Study the drawing (mm; zero at the part's minimum x, y, z) and answer. A direction names the side the tool comes from. Round coordinates to 2 decimals unless told otherwise and drop trailing zeros. Loops run counter-clockwise (first coordinate to the right, second up) from the corner with the lowest first, then second, coordinate; pieces in that order, holes last. Notation, with made-up numbers: M 28,-29 L 78,-29 A21 cw 78,-12 Z; hole C 52,-4.5 d2. An arc over 180 degrees is marked long. Put each result on its own line as item: value. Start each with the question number.
(1) Which of the six approach directions +Z, -Z, +X, -X, +Y, -Y give full straight-line access (tool end or side, diameter ignored) to the marked faces 1 and 2?
(2) Section B-B, the plane x = 28.5 is taken. Determine the outline of the cut face in (y, z).
(3) Section A-A, the plane y = 1.5 is taken. Determine the outline of the cut face in (x, z).
(4) Section C-C, the plane z = 6 is taken. Determine the outline of the cut face in (x, y).
(5) Determine the mould class of the marked faces 3, 4, 5 and 6 for opening direction X: released by +X, released by -X, zero draft, split by the parting line, or undercut.
(6) Section D-D, the plane y = 9 is taken. Determine the outline of the cut face in (x, z), then the cut area to 3 significant figures.
(7) Straight lines are drawn through the part: line 1 (X direction, y = 9.75, z = 41.9); line 2 (Z direction, x = 28.5, y = 10.35); line 3 (X direction, y = 5, z = 37). For each, find the intervals that lie inside material, in ascending order.
(8) Flat-ended cylindrical pins translate along their axes: P1, Ø1.8, axis at x = 3.5, z = 41.9, coming from the +Y side; P2, Ø6, axis at x = 25.5, y = 3.5, coming from the +Z side; P3, Ø1.5, axis at x = 20.5, y = 4, coming from the -Z side; P4, Ø4.5, axis at x = 16, z = 28.5, coming from the -Y side. Find the tip coordinate at first contact, or state that the pin passes through.
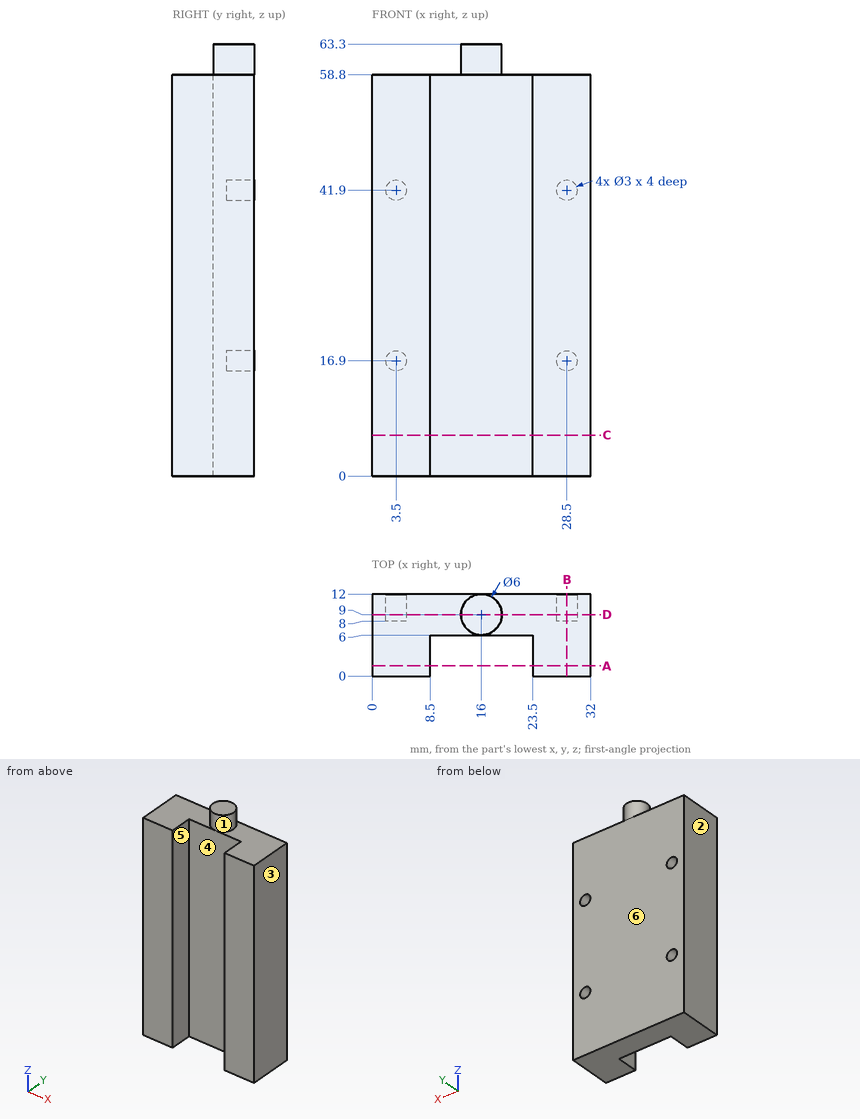
Recorded:
1. face 1: +Z
1. face 2: +Z, -Z, -X, +Y, -Y
2. outline: M 0,0 L 12,0 L 12,15.4 L 8,15.4 L 8,18.4 L 12,18.4 L 12,40.4 L 8,40.4 L 8,43.4 L 12,43.4 L 12,58.8 L 0,58.8 Z
3. outline: M 0,0 L 8.5,0 L 8.5,58.8 L 0,58.8 Z; M 23.5,0 L 32,0 L 32,58.8 L 23.5,58.8 Z
4. outline: M 0,0 L 8.5,0 L 8.5,6 L 23.5,6 L 23.5,0 L 32,0 L 32,12 L 0,12 Z
5. face 3: released by +X
5. face 4: undercut
5. face 5: undercut
5. face 6: zero draft
6. outline: M 0,0 L 32,0 L 32,58.8 L 19,58.8 L 19,63.3 L 13,63.3 L 13,58.8 L 0,58.8 Z; hole C 3.5,16.9 d3; hole C 3.5,41.9 d3; hole C 28.5,16.9 d3; hole C 28.5,41.9 d3
6. area: 1,880 mm²
7. line 1: x = 0 to 2, 5 to 27, 30 to 32
7. line 2: z = 0 to 15.4, 18.4 to 40.4, 43.4 to 58.8
7. line 3: x = 0 to 8.5, 23.5 to 32
8. P1: stops at y = 8
8. P2: stops at z = 58.8
8. P3: passes through
8. P4: stops at y = 6
